Geometry: final body of the model. Coordinates: model frame, mm. A direction names the side the tool comes from. Round coordinates to 2 decimals unless told otherwise and drop trailing zeros. Loops run counter-clockwise (first coordinate to the right, second up) from the corner with the lowest first, then second, coordinate; pieces in that order, holes last. Notation, with made-up numbers: (50.25, -30) -> (74.25, -30) arc R21 cw to (74.25, -17) -> close; hole circle Ø3 at (-40, -3.75). An arc over 180 degrees is marked (long way). Answer in a Markdown table with one row per item.
Autodesk Inventor part; units mm, degrees
ref_plane "YZ Plane" through (0, 0, 0) normal (1, 0, 0) x (0, 1, 0)
ref_plane "XZ Plane" through (0, 0, 0) normal (0, 1, 0) x (-1, 0, 0)
ref_plane "XY Plane" through (0, 0, 0) normal (0, 0, 1) x (1, 0, 0)
sketch "スケッチ1" plane through (0, 0, 0) normal (0, 0, 1) x (1, 0, 0)
  circle A0 centre (0, 0) radius 40
  dimension "d0" = 80
extrude "押し出し1" add sketch "スケッチ1" along normal blind 60
sketch "スケッチ2" plane through (0, 0, 60) normal (0, 0, 1) x (1, 0, 0)
  circle A0 centre (0, 0) radius 32.5
  dimension "d3" = 65
extrude "押し出し2" cut sketch "スケッチ2" against normal blind 60
sketch "スケッチ3" plane through (0, 0, 0) normal (1, 0, 0) x (0, 1, 0)
  line L0 (40, 0) -> (40, 60)
  line L1 (40, 60) -> (-40, 49.2831)
  line L2 (-40, 0) -> (-40, 60)
  line L3 (40, 60) -> (-40, 60)
  line L4 (40, 60) -> (-40, 60)
  line L5 (-40, 60) -> (-40, 49.2831)
  point P0 (0, 0)
extrude "押し出し3" cut sketch "スケッチ3" against normal mid plane 80
sketch "スケッチ4" plane through (0, 0, 0) normal (0, 0, 1) x (1, 0, 0)
  line L0 (-32.5, -6.5) -> (32.5, -6.5)
  line L1 (32.5, -6.5) -> (32.5, 6.5)
  line L2 (32.5, 6.5) -> (-32.5, 6.5)
  line L3 (-32.5, 6.5) -> (-32.5, -6.5)
  line L4 (-32.5, -6.5) -> (32.5, 6.5) construction
  line L5 (32.5, -6.5) -> (-32.5, 6.5) construction
  point P0 (0, 0)
  dimension "d8" = 13
  dimension "d9" = 65
extrude "押し出し4" add sketch "スケッチ4" along normal blind 3
sketch "スケッチ5" plane through (0, 0, 0) normal (0, 0, -1) x (-1, 0, 0)
  point P0 (0, 0)
  point P1 (-20, 0)
  point P2 (20, 0)
  dimension "d12" = 20
  dimension "d13" = 20
hole "穴1" at (20, 0, 0) at (-20, 0, 0) direction (0, 0, 1) diameter 3.2 depth 15 tip angle 118
sketch "スケッチ6" plane through (0, 0, 0) normal (0, 0, -1) x (-1, 0, 0)
  point P0 (0, 0)
  point P1 (0, 0)
hole "穴2" at (0, 0, 0) direction (0, 0, 1) diameter 1.5 depth 15 tip angle 118
sketch "スケッチ7" plane through (0, 0, 0) normal (0, 0, -1) x (-1, 0, 0)
  point P0 (0, 0)
  point P1 (-8.3, 0)
  point P2 (8.3, 0)
  dimension "d28" = 8.3
  dimension "d29" = 8.3
hole "穴3" at (8.3, 0, 0) at (-8.3, 0, 0) direction (0, 0, 1) diameter 3.2 depth 8.8 tip angle 118
properties part number "20220612_仮筒"
Item 1: Line query: probe 1 along X at (y, z) = (0, 1); probe 2 along Y at (x, z) = (0, 1.35); probe 3 along Y at (x, z) = (8.3, 0.95). Output: solid intervals per line, ascending. Write a range as [from, to].
Answer:
| item | result |
|---|---|
| probe 1 | x = [-40, -21.6], [-18.4, -9.9], [-6.7, -0.75], [0.75, 6.7], [9.9, 18.4], [21.6, 40] |
| probe 2 | y = [-40, -32.5], [-6.5, -0.75], [0.75, 6.5], [32.5, 40] |
| probe 3 | y = [-39.13, -31.42], [-6.5, -1.6], [1.6, 6.5], [31.42, 39.13] |
Item 2: Draft query along X for faces 4 (the face through (32.779, 0.187, 54.667)), 5 (the face through (-8.67, 39.05, 29.58)), 6 (the face through (0, 6.5, 1)). Return one class per face: pulls with the +X half, pulls with the -X half, needs draft (parallel to the pull), parting line crosses it, or undercut.
Answer:
| item | result |
|---|---|
| face 4 | needs draft |
| face 5 | parting line crosses it |
| face 6 | undercut |
Item 3: Cut plane A-A (x = 8.3). Output: boundary loops of the cut face in (y, z).
Answer:
| item | result |
|---|---|
| outline | (-39.13, 0) -> (-31.42, 0) -> (-31.42, 50.43) -> (-39.13, 49.4) -> close; (-6.5, 0) -> (-1.6, 0) -> (-1.6, 3) -> (-6.5, 3) -> close; (1.6, 0) -> (6.5, 0) -> (6.5, 3) -> (1.6, 3) -> close; (31.42, 0) -> (39.13, 0) -> (39.13, 59.88) -> (31.42, 58.85) -> close |
Item 4: Cut plane B-B (y = -28.5). Output: boundary loops of the cut face in (x, z).
Answer:
| item | result |
|---|---|
| outline | (-28.07, 0) -> (-15.62, 0) -> (-15.62, 50.82) -> (-28.07, 50.82) -> close; (15.62, 0) -> (28.07, 0) -> (28.07, 50.82) -> (15.62, 50.82) -> close |
Item 5: Reachability of faces 1 (the face through (0, 2, 3)), 2 (the face through (3, 0, 0)), 3 (the face through (0, -6.5, 1)) from +Z, -Z, +X, -X, +Y, -Y: full face, straight path, thin tool, end or side. Return the list, or none.
Answer:
| item | result |
|---|---|
| face 1 | +Z |
| face 2 | -Z, +X, -X, +Y, -Y |
| face 3 | +Z, -Z |
Item 6: Cut plane C-C (z = 18). Output: boundary loops of the cut face in (x, y).
Answer:
| item | result |
|---|---|
| outline | circle Ø80 at (0, 0); hole circle Ø65 at (0, 0) |
Item 7: Pin query (flat end, axial travel): pin 1 Ø5 at (y, z) = (17, 25.5) entering from -X; pin 2 Ø2 at (y, z) = (-28.5, 20.5) entering from +X; pin 3 Ø0.9 at (x, z) = (1, 1) entering from -Y; pin 4 Ø3 at (x, y) = (20, 0) entering from +Z. Return the tip coordinate at first contact, or that it passes through.
Answer:
| item | result |
|---|---|
| pin 1 | stops at x = -37.28 |
| pin 2 | stops at x = 29.05 |
| pin 3 | stops at y = -40 |
| pin 4 | passes through |
Item 8: Cut plane D-D (y = 16). Output: boundary loops of the cut face in (x, z).
Answer:
| item | result |
|---|---|
| outline | (-36.66, 0) -> (-28.29, 0) -> (-28.29, 56.78) -> (-36.66, 56.78) -> close; (28.29, 0) -> (36.66, 0) -> (36.66, 56.78) -> (28.29, 56.78) -> close |
